```python
from build123d import *

# Parameters (mm, degrees)
SKETCH1_R      = 2.6035
EXTRUDE1_DEPTH = 25.4


with BuildPart() as part:
    # Sketch1 → Extrude1 (new body)
    with BuildSketch(Plane.XY):
        with BuildLine():
            Line((813.038976674, 579.290424026), (813.038976674, 582.236824026))
            ThreePointArc((813.038976674, 582.236824026), (812.530976674, 582.744824026), (813.038976674, 583.252824026))
            Line((813.038976674, 583.252824026), (813.038976674, 584.484724026))
            ThreePointArc((813.038976674, 584.484724026), (811.934076674, 585.589624026), (810.829176674, 584.484724026))
            Line((810.829176674, 584.484724026), (810.829176674, 582.435874947))
            ThreePointArc((810.829176674, 582.435874947), (810.182743454, 581.495163196), (809.057340701, 581.685644565))
            Line((809.057340701, 581.685644565), (805.773323088, 584.969563516))
            ThreePointArc((805.773323088, 584.969563516), (805.085045004, 585.999619341), (804.843353394, 587.214661271))
            Line((804.843353394, 587.214661271), (804.843353394, 590.467068589))
            ThreePointArc((804.843353394, 590.467068589), (805.085043572, 591.682107061), (805.773317796, 592.712161052))
            Line((805.773317796, 592.712161052), (809.057121325, 595.995881407))
            ThreePointArc((809.057121325, 595.995881407), (810.18544278, 596.185153907), (810.829176674, 595.239352628))
            Line((810.829176674, 595.239352628), (810.829176674, 593.196924026))
            ThreePointArc((810.829176674, 593.196924026), (811.934076674, 592.092024026), (813.038976674, 593.196924026))
            Line((813.038976674, 593.196924026), (813.038976674, 594.428824026))
            ThreePointArc((813.038976674, 594.428824026), (812.530976674, 594.936824026), (813.038976674, 595.444824026))
            Line((813.038976674, 595.444824026), (813.038976674, 598.391224026))
            ThreePointArc((813.038976674, 598.391224026), (812.530976674, 598.899224026), (813.038976674, 599.407224026))
            Line((813.038976674, 599.407224026), (813.038976674, 599.432624026))
            ThreePointArc((813.038976674, 599.432624026), (812.42149919, 600.923346542), (810.930776674, 601.540824026))
            Line((810.930776674, 601.540824026), (810.905376674, 601.540824026))
            ThreePointArc((810.905376674, 601.540824026), (810.397376674, 601.032824026), (809.889376674, 601.540824026))
            Line((809.889376674, 601.540824026), (806.942976674, 601.540824026))
            ThreePointArc((806.942976674, 601.540824026), (806.434976674, 601.032824026), (805.926976674, 601.540824026))
            Line((805.926976674, 601.540824026), (804.695076674, 601.540824026))
            ThreePointArc((804.695076674, 601.540824026), (803.590176674, 600.435924026), (804.695076674, 599.331024026))
            Line((804.695076674, 599.331024026), (806.743925753, 599.331024026))
            ThreePointArc((806.743925753, 599.331024026), (807.684637504, 598.684590806), (807.494156135, 597.559188053))
            Line((807.494156135, 597.559188053), (804.210237184, 594.27517044))
            ThreePointArc((804.210237184, 594.27517044), (803.180181359, 593.586892356), (801.965139429, 593.345200745))
            Line((801.965139429, 593.345200745), (798.712732111, 593.345200745))
            ThreePointArc((798.712732111, 593.345200745), (797.497693639, 593.586890924), (796.467639648, 594.275165148))
            Line((796.467639648, 594.275165148), (793.183919293, 597.558968677))
            ThreePointArc((793.183919293, 597.558968677), (792.994646793, 598.687290132), (793.940448072, 599.331024026))
            Line((793.940448072, 599.331024026), (795.982876674, 599.331024026))
            ThreePointArc((795.982876674, 599.331024026), (797.087776674, 600.435924026), (795.982876674, 601.540824026))
            Line((795.982876674, 601.540824026), (794.750976674, 601.540824026))
            ThreePointArc((794.750976674, 601.540824026), (794.242976674, 601.032824026), (793.734976674, 601.540824026))
            Line((793.734976674, 601.540824026), (790.788576674, 601.540824026))
            ThreePointArc((790.788576674, 601.540824026), (790.280576674, 601.032824026), (789.772576674, 601.540824026))
            Line((789.772576674, 601.540824026), (789.747176674, 601.540824026))
            ThreePointArc((789.747176674, 601.540824026), (788.256454158, 600.923346542), (787.638976674, 599.432624026))
            Line((787.638976674, 599.432624026), (787.638976674, 599.407224026))
            ThreePointArc((787.638976674, 599.407224026), (788.146976674, 598.899224026), (787.638976674, 598.391224026))
            Line((787.638976674, 598.391224026), (787.638976674, 595.444824026))
            ThreePointArc((787.638976674, 595.444824026), (788.146976674, 594.936824026), (787.638976674, 594.428824026))
            Line((787.638976674, 594.428824026), (787.638976674, 593.196924026))
            ThreePointArc((787.638976674, 593.196924026), (788.743876674, 592.092024026), (789.848776674, 593.196924026))
            Line((789.848776674, 593.196924026), (789.848776674, 595.245773105))
            ThreePointArc((789.848776674, 595.245773105), (790.495209894, 596.186484856), (791.620612647, 595.996003487))
            Line((791.620612647, 595.996003487), (794.90463026, 592.712084536))
            ThreePointArc((794.90463026, 592.712084536), (795.592908344, 591.682028711), (795.834599954, 590.466986781))
            Line((795.834599954, 590.466986781), (795.834599954, 587.214579463))
            ThreePointArc((795.834599954, 587.214579463), (795.592909776, 585.999540991), (794.904635552, 584.969487))
            Line((794.904635552, 584.969487), (791.620832022, 581.685766645))
            ThreePointArc((791.620832022, 581.685766645), (790.492510568, 581.496494145), (789.848776674, 582.442295424))
            Line((789.848776674, 582.442295424), (789.848776674, 584.484724026))
            ThreePointArc((789.848776674, 584.484724026), (788.743876674, 585.589624026), (787.638976674, 584.484724026))
            Line((787.638976674, 584.484724026), (787.638976674, 583.252824026))
            ThreePointArc((787.638976674, 583.252824026), (788.146976674, 582.744824026), (787.638976674, 582.236824026))
            Line((787.638976674, 582.236824026), (787.638976674, 579.290424026))
            ThreePointArc((787.638976674, 579.290424026), (788.146976674, 578.782424026), (787.638976674, 578.274424026))
            Line((787.638976674, 578.274424026), (787.638976674, 578.249024026))
            ThreePointArc((787.638976674, 578.249024026), (788.256454158, 576.75830151), (789.747176674, 576.140824026))
            Line((789.747176674, 576.140824026), (789.772576674, 576.140824026))
            ThreePointArc((789.772576674, 576.140824026), (790.280576674, 576.648824026), (790.788576674, 576.140824026))
            Line((790.788576674, 576.140824026), (793.734976674, 576.140824026))
            ThreePointArc((793.734976674, 576.140824026), (794.242976674, 576.648824026), (794.750976674, 576.140824026))
            Line((794.750976674, 576.140824026), (795.982876674, 576.140824026))
            ThreePointArc((795.982876674, 576.140824026), (797.087776674, 577.245724026), (795.982876674, 578.350624026))
            Line((795.982876674, 578.350624026), (793.934027595, 578.350624026))
            ThreePointArc((793.934027595, 578.350624026), (792.993315844, 578.997057246), (793.183797213, 580.122459999))
            Line((793.183797213, 580.122459999), (796.467716164, 583.406477612))
            ThreePointArc((796.467716164, 583.406477612), (797.497771989, 584.094755696), (798.712813919, 584.336447306))
            Line((798.712813919, 584.336447306), (801.965221237, 584.336447306))
            ThreePointArc((801.965221237, 584.336447306), (803.180259709, 584.094757128), (804.2103137, 583.406482904))
            Line((804.2103137, 583.406482904), (807.494034055, 580.122679374))
            ThreePointArc((807.494034055, 580.122679374), (807.683306555, 578.99435792), (806.737505276, 578.350624026))
            Line((806.737505276, 578.350624026), (804.695076674, 578.350624026))
            ThreePointArc((804.695076674, 578.350624026), (803.590176674, 577.245724026), (804.695076674, 576.140824026))
            Line((804.695076674, 576.140824026), (805.926976674, 576.140824026))
            ThreePointArc((805.926976674, 576.140824026), (806.434976674, 576.648824026), (806.942976674, 576.140824026))
            Line((806.942976674, 576.140824026), (809.889376674, 576.140824026))
            ThreePointArc((809.889376674, 576.140824026), (810.397376674, 576.648824026), (810.905376674, 576.140824026))
            Line((810.905376674, 576.140824026), (810.930776674, 576.140824026))
            ThreePointArc((810.930776674, 576.140824026), (812.42149919, 576.75830151), (813.038976674, 578.249024026))
            Line((813.038976674, 578.249024026), (813.038976674, 578.274424026))
            ThreePointArc((813.038976674, 578.274424026), (812.530976674, 578.782424026), (813.038976674, 579.290424026))
        make_face()
        with Locations((800.338976674, 588.840824026)):
            Circle(SKETCH1_R, mode=Mode.SUBTRACT)
    extrude(amount=-EXTRUDE1_DEPTH)


solid = part.part
```
Check sheet for the modelled part. Datum: model origin and axes. Units: mm. A direction names the side the tool comes from. Coordinates: 2 decimals unless noted, no trailing zeros. Write each loop counter-clockwise with the first axis right and the second up, starting at its lowest first coordinate (ties: lowest second). Pieces come first, ordered by that corner, then holes. Notation, with made-up numbers: M -25,10 L -4,10 A30 cw -4,37 Z; hole C 45.5,-19.5 d4. An arc over 180 degrees is marked long. Use one line per item in the form item = value.
Item 1: Sectioned sample at A-A, the plane x = 810.25. Record the cut outline in (y, z) (3 decimals).
Answer below:
outline = M 576.627,-25.4 L 581.526,-25.4 L 581.526,0 L 576.627,0 Z; M 596.155,-25.4 L 601.055,-25.4 L 601.055,0 L 596.155,0 Z
Item 2: Set-up check for faces 1 (the face through (790.51, 581.49, -12.52)), 2 (the face through (813.039, 594, -13)): record each of +Z, -Z, +X, -X, +Y, -Y from which the full face is reachable in a straight line by a thin tool's end or side.
Answer below:
face_1 = +Z, -Z
face_2 = +Z, -Z, +X, +Y, -Y
Item 3: Material ranges on L1, parallel to X at y = 592.25, z = -9.25; L2, parallel to X at y = 589, z = -3; L3, parallel to Y at x = 806, z = -24, recorded low to high. Write a range as from..to.
Answer below:
L1 = 788.17..789.31, 795.29..805.39, 811.36..812.5
L2 = 795.83..797.74, 802.94..804.84
L3 = 576.4..578.35, 581.62..584.74, 592.94..596.06, 599.33..601.28
Item 4: Gauge pin test, flat ends, axial feed: pin 1 Ø2 at (x, y) = (796.5, 597.5) entering from +Z; pin 2 Ø1.6 at (y, z) = (588, -8) entering from -X; pin 3 Ø2.5 at (x, z) = (800, -11.5) entering from -Y; pin 4 Ø3.5 at (x, z) = (800, -16) entering from +Y. Record the tip position at first contact, or that the pin passes through.
Answer below:
pin_1 = through
pin_2 = 795.83
pin_3 = 584.34
pin_4 = 593.38
Item 5: Release check for a two-part mould opening along Y. For faces 3 (the face through (813.039, 584, -13)), 4 (the face through (800, 593.345, -13)), 5 (the face through (810.829, 583, -13)), 6 (the face through (803.59, 577.27, -12.52)) record: pulls with the +Y half, pulls with the -Y half, needs draft (parallel to the pull), parting line crosses it, or undercut.
Answer below:
face_3 = needs draft
face_4 = pulls with the +Y half
face_5 = undercut
face_6 = undercut
Item 6: Sectioned sample at B-B, the plane y = 580.5. Record the cut outline in (x, z), and give its area (3 significant figures).
Answer below:
outline = M 787.64,-25.4 L 793.56,-25.4 L 793.56,0 L 787.64,0 Z; M 807.12,-25.4 L 813.04,-25.4 L 813.04,0 L 807.12,0 Z
area = 301 mm^2
